```python
from build123d import *

# Parameters (mm, degrees)
SKETCH1_R           = 5
SKETCH1_R_2         = 1.75
BOSS_EXTRUDE1_DEPTH = 5
BOSS_EXTRUDE2_START = -5
BOSS_EXTRUDE2_DEPTH = 5


with BuildPart() as part:
    # Sketch1 → Boss-Extrude1 (new body)
    # profile 1 of 3: a face of its own
    with BuildSketch(Plane(origin=(0, 0, 0), x_dir=(0, 0, -1), z_dir=(1, 0, 0))):
        with Locations((5, 5)):
            Circle(SKETCH1_R)
        with Locations((5, 5)):
            Circle(SKETCH1_R_2, mode=Mode.SUBTRACT)
    # profile 2 of 3: a face of its own
    with BuildSketch(Plane(origin=(0, 0, 0), x_dir=(0, 0, -1), z_dir=(1, 0, 0))):
        with BuildLine():
            Line((27, 10), (5, 10))
            ThreePointArc((5, 10), (8.535533906, 8.535533906), (10, 5))
            ThreePointArc((10, 5), (8.535533906, 1.464466094), (5, 0))
            Line((5, 0), (27, 0))
            ThreePointArc((27, 0), (22, 5), (27, 10))
        make_face()
    # profile 3 of 3: a face of its own
    with BuildSketch(Plane(origin=(0, 0, 0), x_dir=(0, 0, -1), z_dir=(1, 0, 0))):
        with Locations((27, 5)):
            Circle(SKETCH1_R)
        with Locations((27, 5)):
            Circle(SKETCH1_R_2, mode=Mode.SUBTRACT)
    extrude(amount=BOSS_EXTRUDE1_DEPTH)

    # Sketch2 → Boss-Extrude2 (add)
    with BuildSketch(Plane(origin=(5, 0, 0), x_dir=(0, 0, -1), z_dir=(1, 0, 0)).offset(BOSS_EXTRUDE2_START)):
        with BuildLine():
            Line((65.975697465, 13.736161147), (64.607616892, 17.49493163))
            add(Edge.make_bspline(
                [(14, 10), (22.729658928, 11.165748207), (34.565066024, 15.059942726), (50.556554523, 24.001893285), (64.607616892, 17.49493163)],
                knots=[0, 0, 0, 0, 0.349113353, 1, 1, 1, 1], degree=3))
            Line((14, 10), (27, 10))
            ThreePointArc((27, 10), (31.871850324, 6.124755272), (29.191855734, 0.506029769))
            Line((29.191855734, 0.506029769), (38.089916792, 4.845904122))
            ThreePointArc((38.089916792, 4.845904122), (46.993994408, 12.1595138), (58.458156499, 11))
            Line((58.458156499, 11), (65.975697465, 13.736161147))
        make_face()
    extrude(amount=BOSS_EXTRUDE2_DEPTH)


solid = part.part
```
Geometry check sheet. Reference: the model listing, model coordinates, mm. A direction names the side the tool comes from. Coordinates: 2 decimals unless noted, no trailing zeros. Loops run counter-clockwise (first coordinate to the right, second up) from the corner with the lowest first, then second, coordinate; pieces in that order, holes last. Notation, with made-up numbers: (56.25, 26) - (68.25, 26) arc R23 ccw to (68.25, 43) - close; hole circle Ø7 at (-4.75, -23.5). An arc over 180 degrees is marked (long way). One line per item, written item: value. Start each with the question number.
(1) Depth check by flat-ended pin: P1, Ø3, axis at x = 4, y = 16.5, coming from the -Z side; P2, Ø3, axis at x = 2.5, y = 5.5, coming from the -Z side; P3, Ø2, axis at y = 5, z = -5, coming from the +X side (1 decimal). Enter the tip coordinate at first touch or a pass-through.
(2) Mould release check, pull along Y, two halves, no side actions. Record for faces 3 (the cylindrical face through (2.46, 3.94, -3.61)), 4 (the flat face through (2, 0, -16)), 5 (the cylindrical face through (2.46, 5.08, -25.25)), 6 (the flat face through (0, 10, -33)): released by +Y, released by -Y, zero draft, split by the parting line, or undercut.
(3) Cross-section at A-A on y = 5.75. Enter the section's corners in (x, z), plus the area to 3 significant figures.
(4) Material ranges on line 1 (Y direction, x = 2.2, z = -5); line 2 (Y direction, x = 3.5, z = -27); line 3 (Y direction, x = 2, z = -13), recorded low to high. Write a range as [from, to].
(5) Tool access check on faces 1 (the flat face through (2, 10, -10)), 2 (the flat face through (5, 10, -33)). Record the directions out of +Z, -Z, +X, -X, +Y, -Y that give a thin tool (end or side, any length) a straight path to the whole face; none if there is none.
Results below:
1. P1: stops at z = -65.52
1. P2: stops at z = -39.48
1. P3: passes through
2. face 3: undercut
2. face 4: released by -Y
2. face 5: undercut
2. face 6: zero draft
3. outline: (0, -38.61) - (5, -38.61) - (5, -28.58) - (0, -28.58) - close; (0, -25.42) - (5, -25.42) - (5, -6.58) - (0, -6.58) - close; (0, -3.42) - (5, -3.42) - (5, -0.06) - (0, -0.06) - close
3. area: 161 mm2
4. line 1: y = [0, 3.25], [6.75, 10]
4. line 2: y = [0, 3.25], [6.75, 12.77]
4. line 3: y = [0, 10]
5. face 1: +Z, +X, -X, +Y
5. face 2: +Z, -Z, +X, +Y, -Y
